from build123d import *

# Parameters (mm, degrees)
SKETCH1_R           = 46.99
BOSS_EXTRUDE1_DEPTH = 3.175
SKETCH2_R           = 14.351
CUT_EXTRUDE1_DEPTH  = 3.175
CUT_EXTRUDE2_DEPTH  = 7.62
SKETCH6_R           = 31.75
CUT_EXTRUDE3_DEPTH  = 5.08


with BuildPart() as part:
    # Sketch1 → Boss-Extrude1 (new body)
    with BuildSketch(Plane(origin=(0, 0, 0), x_dir=(1, 0, 0), z_dir=(0, 1, 0))):
        with Locations(Location((0, 0, 0), (0, 0, 270))):
            Circle(SKETCH1_R)
    extrude(amount=BOSS_EXTRUDE1_DEPTH)

    # Sketch2 → Cut-Extrude1 (cut)
    with BuildSketch(Plane(origin=(0, 3.175, 0), x_dir=(1, 0, 0), z_dir=(0, 1, 0))):
        with Locations(Location((0, 0, 0), (0, 0, 270))):
            Circle(SKETCH2_R)
    extrude(amount=-CUT_EXTRUDE1_DEPTH, mode=Mode.SUBTRACT)

    # Sketch5 → Cut-Extrude2 (cut)
    with BuildSketch(Plane(origin=(0, 3.175, 0), x_dir=(1, 0, 0), z_dir=(0, 1, 0))):
        with BuildLine():
            Line((3.175, 13.995376951), (3.175, 44.45))
            Line((3.175, 44.45), (-3.175, 44.45))
            Line((-3.175, 44.45), (-3.175, 13.995376951))
            ThreePointArc((-3.175, 13.995376951), (0, 14.351), (3.175, 13.995376951))
        make_face()
        with BuildLine():
            Line((3.175, -44.45), (3.175, -13.995376951))
            ThreePointArc((3.175, -13.995376951), (0, -14.351), (-3.175, -13.995376951))
            Line((-3.175, -13.995376951), (-3.175, -44.45))
            Line((-3.175, -44.45), (3.175, -44.45))
        make_face()
        with BuildLine():
            ThreePointArc((-13.995376951, -3.175), (-14.351, 0), (-13.995376951, 3.175))
            Line((-13.995376951, 3.175), (-44.45, 3.175))
            Line((-44.45, 3.175), (-44.45, -3.175))
            Line((-44.45, -3.175), (-13.995376951, -3.175))
        make_face()
        with BuildLine():
            Line((44.45, 3.175), (13.995376951, 3.175))
            ThreePointArc((13.995376951, 3.175), (14.261817129, 1.597427053), (14.351, 0))
            ThreePointArc((14.351, 0), (14.261817129, -1.597427053), (13.995376951, -3.175))
            Line((13.995376951, -3.175), (44.45, -3.175))
            Line((44.45, -3.175), (44.45, 3.175))
        make_face()
    extrude(amount=-CUT_EXTRUDE2_DEPTH, mode=Mode.SUBTRACT)

    # Sketch6 → Cut-Extrude3 (cut)
    with BuildSketch(Plane(origin=(0, 3.175, 0), x_dir=(1, 0, 0), z_dir=(0, 1, 0))):
        Circle(SKETCH6_R)
    extrude(amount=-CUT_EXTRUDE3_DEPTH, mode=Mode.SUBTRACT)


solid = part.part
Read the model definition and answer for the solid it produces. Units are mm, in the model's axes. A direction names the side the tool comes from. Coordinates: 2 decimals unless noted, no trailing zeros. Order: outer loops, then holes, each group sorted by start corner. A loop starts at its lowest first (then second) coordinate and runs counter-clockwise, first axis right, second up. Notation, with made-up numbers: M 73,7.25 L 77,7.25 A18 cw 77,14.25 Z; hole C 15,-1.75 d11. An arc over 180 degrees is marked long. Put each result on its own line as item: value. Start each with the question number.
Item 1: The mould has two halves that part along Z. Classify faces 1 (the face through (-45.87, 1.57, -10.19)), 2 (the face through (3.175, 2, -38)), 3 (the face through (-31, 3.175, 10)): +Z half, -Z half, draft (parallel to the pull), parting line (faces both ways), or undercut.
Item 2: For faces 4 (the face through (-31, 0, 10)), 5 (the face through (0, 2, -44.45)), determine the directions among +Z, -Z, +X, -X, +Y, -Y from which every point of the face is accessible in a straight line to the end or side of a thin tool.
Item 3: Section C-C, the plane y = 2.65 is taken. Determine the outline of the cut face in (x, z) (3 decimals), plus the area to 3 significant figures.
Item 4: Consider probe 1 along Z at (x, y) = (-35, 2.65) (3 decimals); probe 2 along X at (y, z) = (0.5, 37) (3 decimals); probe 3 along X at (y, z) = (3, 20.5). Determine where each line is inside the solid, lowest interval first. Write a range as [from, to].
Item 5: Section A-A, the plane x = 0 is taken. Determine the outline of the cut face in (y, z) (3 decimals), plus the area to 3 significant figures.
Item 6: Given pin 1 Ø1 at (y, z) = (2, -1) entering from -X; pin 2 Ø1 at (x, y) = (-1, 1.5) entering from -Z; pin 3 Ø1.6 at (x, y) = (-38.5, 2) entering from +Z, each flat-ended and moving along its own axis, determine where each tip first touches the part or whether it passes through.
Item 7: Section B-B, the plane z = 0 is taken. Determine the outline of the cut face in (x, y) (3 decimals).
Computed:
1. face 1: parting line
1. face 2: undercut
1. face 3: draft
2. face 4: +Z, -Z, +X, -X, -Y
2. face 5: +Y, -Y
3. outline: C 0,0 d93.98; hole M -44.45,-3.175 L -31.591,-3.175 A31.75 ccw -3.175,-31.591 L -3.175,-44.45 L 3.175,-44.45 L 3.175,-31.591 A31.75 ccw 31.591,-3.175 L 44.45,-3.175 L 44.45,3.175 L 31.591,3.175 A31.75 ccw 3.175,31.591 L 3.175,44.45 L -3.175,44.45 L -3.175,31.591 A31.75 ccw -31.591,3.175 L -44.45,3.175 Z
3. area: 3,450 mm2
4. probe 1: z = [-31.354, -3.175], [3.175, 31.354]
4. probe 2: x = [-28.967, -3.175], [3.175, 28.967]
4. probe 3: x = [-42.28, -24.24], [24.24, 42.28]
5. outline: M 0,-46.99 L 3.175,-46.99 L 3.175,-44.45 L 0,-44.45 Z; M 0,44.45 L 3.175,44.45 L 3.175,46.99 L 0,46.99 Z
5. area: 16.1 mm2
6. pin 1: stops at x = -46.99
6. pin 2: stops at z = -46.99
6. pin 3: stops at z = 28.05
7. outline: M -46.99,0 L -44.45,0 L -44.45,3.175 L -46.99,3.175 Z; M 44.45,0 L 46.99,0 L 46.99,3.175 L 44.45,3.175 Z
